Here's how the part is built. I have some questions about the finished solid (model axes, mm). Round coordinates to 2 decimals unless told otherwise and drop trailing zeros. Order: outer loops, then holes, each group sorted by start corner. A loop starts at its lowest first (then second) coordinate and runs counter-clockwise, first axis right, second up. Notation, with made-up numbers: (72.5, 43.25) -> (104.5, 43.25) arc R22 ccw to (104.5, 74.25) -> close; hole circle Ø2 at (-10.5, 54.25). An arc over 180 degrees is marked (long way). Use a Markdown table: item, result. Add a question column.
from build123d import *

# Parameters (mm, degrees)
SKETCH1_W              = 80
SKETCH1_H              = 80
PCB_DEPTH              = 2
SKETCH2_R              = 1.8
ATTACHMENT_HOLES_DEPTH = 3
LPATTERN1_COUNT        = 2
LPATTERN1_PITCH        = 70
LPATTERN1_COUNT_DIR2   = 2
LPATTERN1_PITCH_DIR2   = 70


with BuildPart() as part:
    # Sketch1 → PCB (new body)
    with BuildSketch(Plane(origin=(0, 0, 0), x_dir=(1, 0, 0), z_dir=(0, 1, 0))):
        with Locations((40, 40)):
            Rectangle(SKETCH1_W, SKETCH1_H)
    extrude(amount=PCB_DEPTH)

    # Sketch2 → Attachment Holes (cut, through all)
    with BuildSketch(Plane(origin=(0, 2, 0), x_dir=(1, 0, 0), z_dir=(0, 1, 0))):
        with Locations((5, 75)):
            Circle(SKETCH2_R)
    attachment_holes = extrude(amount=-ATTACHMENT_HOLES_DEPTH, mode=Mode.SUBTRACT)

    # LPattern1: Attachment Holes 2 × 2
    with Locations(*[(i * LPATTERN1_PITCH, 0, j * LPATTERN1_PITCH_DIR2) for i in range(LPATTERN1_COUNT) for j in range(LPATTERN1_COUNT_DIR2) if (i, j) != (0, 0)]):
        add(attachment_holes, mode=Mode.SUBTRACT)


solid = part.part
(1) I'm going to push flat-ended pins straight in: P1, Ø10, axis at x = 62, z = -14.5, coming from the -Y side; P2, Ø2, axis at x = 5, z = -5, coming from the -Y side. Where does each tip first touch, or does it pass through?
(2) If we mould it in two halves opening along X, with no side actions, what happens to faces 1 (the flat face through (80, 1, -39)), 2 (the flat face through (0, 1, -39)), 3 (the cylindrical face through (73.2, 1.01, -5.08))? For each: pulls with the +X half, pulls with the -X half, needs draft (parallel to the pull), parting line crosses it, or undercut.
(3) Please list where these lines run through material, in increasing order: probe 1 along Z at (x, y) = (5, 0.95); probe 2 along X at (y, z) = (0.85, -5). Write a range as from..to.
(4) I want a section at A-A on z = -75. List the corners of the cut face in (x, y) for me.
(5) I want a section at B-B on x = 5. List the corners of the cut face in (y, z) for me, and give its area (3 significant figures).
Output:
| question | item | result |
|---|---|---|
| 1 | P1 | y = 0 |
| 1 | P2 | through |
| 2 | face 1 | pulls with the +X half |
| 2 | face 2 | pulls with the -X half |
| 2 | face 3 | undercut |
| 3 | probe 1 | -80..-76.8, -73.2..-6.8, -3.2..0 |
| 3 | probe 2 | 0..3.2, 6.8..73.2, 76.8..80 |
| 4 | outline | (0, 0) -> (3.2, 0) -> (3.2, 2) -> (0, 2) -> close; (6.8, 0) -> (73.2, 0) -> (73.2, 2) -> (6.8, 2) -> close; (76.8, 0) -> (80, 0) -> (80, 2) -> (76.8, 2) -> close |
| 5 | outline | (0, -80) -> (2, -80) -> (2, -76.8) -> (0, -76.8) -> close; (0, -73.2) -> (2, -73.2) -> (2, -6.8) -> (0, -6.8) -> close; (0, -3.2) -> (2, -3.2) -> (2, 0) -> (0, 0) -> close |
| 5 | area | 146 mm² |
